Work out the finished part from the listing and answer in its coordinate system (mm). A direction names the side the tool comes from. Round coordinates to 2 decimals unless told otherwise and drop trailing zeros. Loops run counter-clockwise (first coordinate to the right, second up) from the corner with the lowest first, then second, coordinate; pieces in that order, holes last. Notation, with made-up numbers: (-25.75, 54) -> (14.25, 54) arc R38 cw to (14.25, 92) -> close; hole circle Ø9 at (50.25, 38.5). An arc over 180 degrees is marked (long way). Use one line per item in the form item = value.
```python
from build123d import *

# Parameters (mm, degrees)
BOSS_EXTRUDE1_DEPTH = 50.8
SKETCH2_R           = 3.175
CUT_EXTRUDE1_DEPTH  = 4.175
SKETCH3_R           = 3.175
CUT_EXTRUDE2_DEPTH  = 4.175


with BuildPart() as part:
    # Sketch1 → Boss-Extrude1 (new body)
    with BuildSketch(Plane.XY):
        Polygon((0, 0), (25.4, 0), (25.4, 3.175), (3.175, 3.175), (3.175, 25.4), (0, 25.4), align=None)
    extrude(amount=BOSS_EXTRUDE1_DEPTH)

    # Sketch2 → Cut-Extrude1 (cut, through all)
    with BuildSketch(Plane(origin=(3.175, 0, 0), x_dir=(0, 0, -1), z_dir=(1, 0, 0))):
        with Locations((-25.4, 12.7)):
            Circle(SKETCH2_R)
    extrude(amount=-CUT_EXTRUDE1_DEPTH, mode=Mode.SUBTRACT)

    # Sketch3 → Cut-Extrude2 (cut, through all)
    with BuildSketch(Plane(origin=(0, 3.175, 0), x_dir=(1, 0, 0), z_dir=(0, 1, 0))):
        with Locations((12.7, -38.1)):
            Circle(SKETCH3_R)
        with Locations((12.7, -12.7)):
            Circle(SKETCH3_R)
    extrude(amount=-CUT_EXTRUDE2_DEPTH, mode=Mode.SUBTRACT)


solid = part.part
```
(1) Find section A-A, the plane x = 12.7. Write down the section's boundary in (y, z) (3 decimals).
Completed:
outline = (0, 0) -> (3.175, 0) -> (3.175, 9.525) -> (0, 9.525) -> close; (0, 15.875) -> (3.175, 15.875) -> (3.175, 34.925) -> (0, 34.925) -> close; (0, 41.275) -> (3.175, 41.275) -> (3.175, 50.8) -> (0, 50.8) -> close
(2) Find section B-B, the plane z = 25.4. Write down the section's boundary in (x, y) (3 decimals), then the cut area to 3 significant figures.
Completed:
outline = (0, 0) -> (25.4, 0) -> (25.4, 3.175) -> (3.175, 3.175) -> (3.175, 9.525) -> (0, 9.525) -> close; (0, 15.875) -> (3.175, 15.875) -> (3.175, 25.4) -> (0, 25.4) -> close
area = 131 mm2
(3) Given P1, Ø8.5, axis at y = 12.7, z = 25.4, coming from the +X side (3 decimals); P2, Ø11, axis at x = 19.5, z = 24.5, coming from the +Y side (3 decimals), each flat-ended and moving along its own axis, determine where each tip first touches the part or whether it passes through.
Completed:
P1 = 3.175
P2 = 3.175
(4) For a pull along Z with two mould halves and no side action, classify faces 1 (the flat face through (7, 2, 0)), 2 (the cylindrical face through (1.61, 11.48, 22.47)), 3 (the flat face through (0, 13, 31)) as +Z half, -Z half, draft (parallel to the pull), parting line (faces both ways), or undercut.
Completed:
face_1 = -Z half
face_2 = undercut
face_3 = draft
(5) Find section C-C, the plane y = 12.7. Write down the section's boundary in (x, z) (3 decimals).
Completed:
outline = (0, 0) -> (3.175, 0) -> (3.175, 22.225) -> (0, 22.225) -> close; (0, 28.575) -> (3.175, 28.575) -> (3.175, 50.8) -> (0, 50.8) -> close
(6) For faces 4 (the cylindrical face through (12.29, 1.61, 34.95)), 5 (the flat face through (3.175, 17, 25)), determine the directions among +Z, -Z, +X, -X, +Y, -Y from which every point of the face is accessible in a straight line to the end or side of a thin tool.
Completed:
face_4 = +Y, -Y
face_5 = +Z, -Z, +X, +Y
(7) Consider L1, parallel to Z at x = 12.7, y = 1.55 (3 decimals); L2, parallel to Y at x = 2.2, z = 25.4 (3 decimals); L3, parallel to X at y = 21.75, z = 41 (3 decimals). Determine where each line is inside the solid, lowest interval first.
Completed:
L1 = 0 to 9.525, 15.875 to 34.925, 41.275 to 50.8
L2 = 0 to 9.525, 15.875 to 25.4
L3 = 0 to 3.175
(8) Find section D-D, the plane z = 33. Write down the section's boundary in (x, y) (3 decimals).
Completed:
outline = (0, 0) -> (25.4, 0) -> (25.4, 3.175) -> (3.175, 3.175) -> (3.175, 25.4) -> (0, 25.4) -> close
